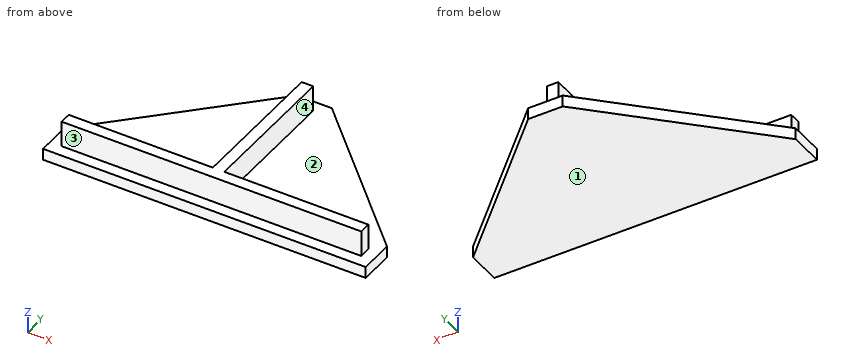
```python
from build123d import *

# Parameters (mm, degrees)
F1_DEPTH = 1.8
F0_W     = 0.8
F0_H     = 0.8
F2_DEPTH = 0.8


with BuildPart() as f1:
    # F0 (on Top) → F1 (new body)
    with BuildSketch(Plane.XY):
        Polygon((-0.4, 10.4), (-0.4, 0.4), (-10.4, 0.4), (-10.4, -0.4), (-0.4, -0.4), (0.4, -0.4), (10.4, -0.4), (10.4, 0.4), (0.4, 0.4), (0.4, 10.4), align=None)
    extrude(amount=F1_DEPTH)

    # F0 (on Top) + F1_face (on face) → F2 (join)
    with BuildSketch(Plane.XY):
        Polygon((-1.2, 11.2), (-11.2, 1.2), (-1.2, 1.2), align=None)
        Polygon((1.2, 1.2), (11.2, 1.2), (1.2, 11.2), align=None)
        Polygon((-10.4, 0.4), (-0.4, 0.4), (-0.4, 10.4), (0.4, 10.4), (0.4, 0.4), (10.4, 0.4), (10.4, -0.4), (0.4, -0.4), (0.4, -1.2), (1.2, -1.2), (11.2, -1.2), (11.2, 1.2), (1.2, 1.2), (1.2, 11.2), (-1.2, 11.2), (-1.2, 1.2), (-11.2, 1.2), (-11.2, -1.2), (-1.2, -1.2), (-0.4, -1.2), (-0.4, -0.4), (-10.4, -0.4), align=None)
        Polygon((-0.4, 10.4), (-0.4, 0.4), (-10.4, 0.4), (-10.4, -0.4), (-0.4, -0.4), (0.4, -0.4), (10.4, -0.4), (10.4, 0.4), (0.4, 0.4), (0.4, 10.4), align=None)
        with Locations((0, -0.8)):
            Rectangle(F0_W, F0_H)
    with BuildSketch(Plane(origin=(0, 1.7532467532, 1.8), x_dir=(1, 0, 0), z_dir=(0, 0, 1))):
        Polygon((0.4, -1.3532467532), (0.4, 8.6467532468), (-0.4, 8.6467532468), (-0.4, -1.3532467532), (-10.4, -1.3532467532), (-10.4, -2.1532467532), (10.4, -2.1532467532), (10.4, -1.3532467532), align=None)
    extrude(amount=-F2_DEPTH)


solid = f1.part
```
Model file for the job. Use its own axes, mm. Face numbers are marked on the shaded views. A direction names the side the tool comes from. Round coordinates to 2 decimals unless told otherwise and drop trailing zeros. Loops run counter-clockwise (first coordinate to the right, second up) from the corner with the lowest first, then second, coordinate; pieces in that order, holes last. Notation, with made-up numbers: M 18,53 L 45,53 A24 ccw 45,85 Z; hole C -35.75,34 d5. An arc over 180 degrees is marked long. Put each result on its own line as item: value. Start each with the question number.
Item 1: 3-axis set-ups, long thin cutter, end or side, ignore diameter. For the marked faces 1, 2, 3 and 4: which of +Z, -Z, +X, -X, +Y, -Y reach the whole face in a straight line?
Item 2: Cut at B-B (x = 9.5). List the corners of the cut face in (y, z), then the cut area to 3 significant figures.
Item 3: Drill centre lines: line 1 along Y through (x, z) = (3.5, 1.6); line 2 along Z through (x, y) = (1.25, 4). Where is each one in solid material? Low to high.
Item 4: Drop flat-ended pins along their axis: P1, Ø0.9, axis at y = 4.5, z = 0.5, coming from the +X side; P2, Ø2, axis at x = 4, y = 8.5, coming from the +Z side; P3, Ø1.5, axis at y = 4, z = -0.5, coming from the +X side. Give the stop position or say it passes through.
Item 5: Cut at A-A (y = 3.25). List the corners of the cut face in (x, z).
Item 6: Cut at C-C (z = -0.25). List the corners of the cut face in (x, y), then the cut area to 3 significant figures.
Answer block:
1. face 1: -Z, +X, -X, +Y, -Y
1. face 2: +Z
1. face 3: +Z, +X, -X, -Y
1. face 4: +Z, +X, +Y
2. outline: M -1.2,-0.8 L 2.9,-0.8 L 2.9,0 L 0.4,0 L 0.4,1.8 L -0.4,1.8 L -0.4,0 L -1.2,0 Z
2. area: 4.72 mm2
3. line 1: -0.4 to 0.4
3. line 2: -0.8 to 0
4. P1: x = 0.4
4. P2: z = 0
4. P3: x = 9.15
5. outline: M -9.15,-0.8 L 9.15,-0.8 L 9.15,0 L 0.4,0 L 0.4,1.8 L -0.4,1.8 L -0.4,0 L -9.15,0 Z
6. outline: M -11.2,-1.2 L 11.2,-1.2 L 11.2,1.2 L 1.2,11.2 L -1.2,11.2 L -11.2,1.2 Z
6. area: 178 mm2
